Build history of the part. All positions in model axes, mm. Face numbers are marked on the shaded views. A direction names the side the tool comes from. Give positions to 0.01 mm unless a question says otherwise; leave off trailing zeros. Order: outer loops, then holes, each group sorted by start corner. A loop starts at its lowest first (then second) coordinate and runs counter-clockwise, first axis right, second up. Notation, with made-up numbers: (8.25, 3) - (17.25, 3) arc R19 ccw to (17.25, 24) - close; hole circle Ø9 at (-16, 42). An arc over 180 degrees is marked (long way). Write each question's results on one line, items separated by ' | '. Start each with the question number.
1) Drill centre lines: line 1 along Z through (x, y) = (-20, 21); line 2 along Y through (x, z) = (-25, 21.5); line 3 along Z through (x, y) = (-12, 13.5). Where is each one in solid material? Low to high. Write a range as from..to.
2) Cut at A-A on y = 19. List the corners of the cut face in (x, z), plus the area to 4 significant figures.
3) Two-plate mould, pull along Y, no slides. Class the marked faces 3, 4 and 5: +Y half, -Y half, draft (parallel to the pull), parting line (faces both ways), or undercut.
4) Cut at C-C on x = -12.5. List the corners of the cut face in (y, z).
5) Cut at D-D on x = -28. List the corners of the cut face in (y, z).
6) Tool access for the marked faces 1 and 2: list every direction of +Z, -Z, +X, -X, +Y, -Y with a clear straight run to the whole face (end or side of a thin tool).
7) Drop flat-ended pins along their axis: pin 1 Ø6 at (x, z) = (-21, 22) entering from +Y; pin 2 Ø6 at (x, z) = (-10, 14.5) entering from +Y; pin 3 Ø11 at (x, y) = (-22, 22.5) entering from +Z. Give the stop position or say it passes through.
8) Cut at B-B on z = 20.5. List the corners of the cut face in (x, y), plus the area to 3 significant figures.
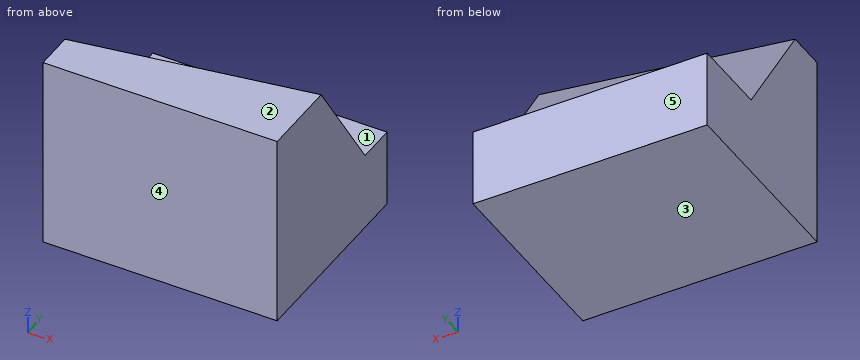
from build123d import *

# Parameters (mm, degrees)
SKETCH1_W           = 30
SKETCH1_H           = 25
BOSS_EXTRUDE1_DEPTH = 25
CUT_EXTRUDE4_DEPTH  = 25


with BuildPart() as part:
    # Sketch1 → Boss-Extrude1 (new body)
    with BuildSketch(Plane.XY):
        with Locations((-15, 12.5)):
            Rectangle(SKETCH1_W, SKETCH1_H)
    extrude(amount=BOSS_EXTRUDE1_DEPTH)

    # 3DSketch1 → Cut-Extrude4 (cut, along a direction that is not the sketch's normal)
    with BuildSketch(Plane(origin=(-30, 15, 10), x_dir=(0.8846517369293828, -0.14744195615489716, 0.4423258684646914), z_dir=(0.13736056394868915, -0.824163383692134, -0.5494422557947564))):
        Polygon((0, 0), (25.802342327, -16.100904646), (33.911649916, 0), (8.109307589, 16.100904646), align=None)
    extrude(amount=-CUT_EXTRUDE4_DEPTH, dir=(0, -1, 0), mode=Mode.SUBTRACT)


solid = part.part
Results:
1) line 1: 0..10 | line 2: 0..8.17 | line 3: 0..16.75
2) outline: (-30, 0) - (0, 0) - (0, 11.5) - (-6, 10) - (-30, 10) - close | area: 304.5 mm^2
3) face 3: draft | face 4: -Y half | face 5: +Y half
4) outline: (0, 0) - (25, 0) - (25, 10) - (17.92, 10) - (7.92, 25) - (0, 25) - close
5) outline: (0, 0) - (25, 0) - (25, 10) - (15.33, 10) - (5.33, 25) - (0, 25) - close
6) face 1: +Z, -X, +Y | face 2: +Z, +X, -X, +Y, -Y
7) pin 1: y = 10.56 | pin 2: y = 17.39 | pin 3: z = 10
8) outline: (-30, 0) - (0, 0) - (0, 13) - (-30, 8) - close | area: 315 mm^2
